Source: CAD feature listing. Evaluate the final solid. Frame: model axes, mm. Face numbers are marked on the shaded views. A direction names the side the tool comes from. Give positions to 0.01 mm unless a question says otherwise; leave off trailing zeros. Order: outer loops, then holes, each group sorted by start corner. A loop starts at its lowest first (then second) coordinate and runs counter-clockwise, first axis right, second up. Notation, with made-up numbers: (57.5, -25) -> (114.5, -25) arc R17 cw to (114.5, 5) -> close; hole circle Ø11 at (-16, -28). An arc over 180 degrees is marked (long way). Answer in a Markdown table with one row per item.
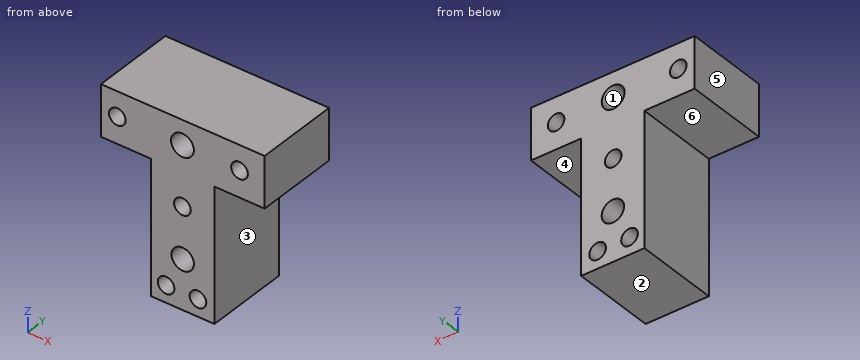
```python
from build123d import *

# Parameters (mm, degrees)
F0_R     = 2.413
F0_R_2   = 3.2512
F0_R_3   = 3.3147
F1_DEPTH = 24.384


with BuildPart() as f1:
    # F0 (on Front) → F1 (new body)
    with BuildSketch(Plane.XZ):
        Polygon((32.9184, 28.943862), (-14.5796, 28.943862), (-14.5796, 14.161062), (0, 14.161062), (0, -24.446938), (18.3388, -24.446938), (18.3388, 14.161062), (32.9184, 14.161062), align=None)
        with Locations((4.317999, -19.524282)):
            Circle(F0_R, mode=Mode.SUBTRACT)
        with Locations((9.143999, -10.159998)):
            Circle(F0_R_2, mode=Mode.SUBTRACT)
        with Locations((13.571819, -19.524282)):
            Circle(F0_R, mode=Mode.SUBTRACT)
        with Locations((9.0678, 4.570901)):
            Circle(F0_R, mode=Mode.SUBTRACT)
        with Locations((-9.830709, 21.781059)):
            Circle(F0_R, mode=Mode.SUBTRACT)
        with Locations((9.0678, 21.808036)):
            Circle(F0_R_3, mode=Mode.SUBTRACT)
        with Locations((25.6286, 21.781059)):
            Circle(F0_R, mode=Mode.SUBTRACT)
    extrude(amount=F1_DEPTH)


solid = f1.part
```
(1) Pull-direction query (X, two-part tool) for the marked faces 1, 2 and 3; classes: +X half, -X half, draft (parallel to the pull), parting line (faces both ways), or undercut.
A:
| item | result |
|---|---|
| face 1 | undercut |
| face 2 | draft |
| face 3 | +X half |
(2) Section query A-A (x = 13). Return the cut outline in (y, z), plus the area to 3 significant figures.
A:
| item | result |
|---|---|
| outline | (-24.38, -24.45) -> (0, -24.45) -> (0, -21.87) -> (-24.38, -21.87) -> close; (-24.38, -17.18) -> (0, -17.18) -> (0, 28.94) -> (-24.38, 28.94) -> close |
| area | 1,190 mm^2 |
(3) Ray query, probe 1 along Z at (x, y) = (9, -21.5); probe 2 along Z at (x, y) = (-10, -5.25); probe 3 along X at (y, z) = (-8, 20). Return the intervals inside material, ascending.
A:
| item | result |
|---|---|
| probe 1 | z = -24.45 to -13.41, -6.91 to 2.16, 6.98 to 18.49, 25.12 to 28.94 |
| probe 2 | z = 14.16 to 19.37, 24.19 to 28.94 |
| probe 3 | x = -14.58 to -11.46, -8.2 to 6.29, 11.85 to 24, 27.26 to 32.92 |
(4) Section query C-C (y = -19.5). Return the cut outline in (x, z), plus the area to 3 significant figures.
A:
| item | result |
|---|---|
| outline | (-14.58, 14.16) -> (0, 14.16) -> (0, -24.45) -> (18.34, -24.45) -> (18.34, 14.16) -> (32.92, 14.16) -> (32.92, 28.94) -> (-14.58, 28.94) -> close; hole circle Ø4.83 at (-9.83, 21.78); hole circle Ø4.83 at (4.32, -19.52); hole circle Ø6.63 at (9.07, 21.81); hole circle Ø6.5 at (9.14, -10.16); hole circle Ø4.83 at (9.07, 4.57); hole circle Ø4.83 at (13.57, -19.52); hole circle Ø4.83 at (25.63, 21.78) |
| area | 1,250 mm^2 |
(5) Access query for the marked faces 4, 5 and 6. Directions: +Z, -Z, +X, -X, +Y, -Y. A direction counts if a zero-diameter tool reaches every point of the face in a straight line with its end or side. Return the directions, or none.
A:
| item | result |
|---|---|
| face 4 | -Z, +X, +Y, -Y |
| face 5 | +Z, -Z, -X, +Y, -Y |
| face 6 | -Z, -X, +Y, -Y |
(6) Section query B-B (z = -11.5). Return the cut outline in (x, y), plus the area to 3 significant figures.
A:
| item | result |
|---|---|
| outline | (0, -24.38) -> (6.18, -24.38) -> (6.18, 0) -> (0, 0) -> close; (12.11, -24.38) -> (18.34, -24.38) -> (18.34, 0) -> (12.11, 0) -> close |
| area | 303 mm^2 |
(7) First-contact query: pin 1 Ø1 at (y, z) = (-12.5, -13) entering from +X; pin 2 Ø10 at (y, z) = (-10.5, -7.5) entering from -X; pin 3 Ø3 at (x, z) = (9.07, 4.57) entering from +Y; pin 4 Ø4.5 at (x, y) = (26.5, -17) entering from -Z. Flat tips, straight axial feed; report the tip coordinate or a pass-through.
A:
| item | result |
|---|---|
| pin 1 | stops at x = 18.34 |
| pin 2 | stops at x = 0 |
| pin 3 | passes through |
| pin 4 | stops at z = 14.16 |
(8) Section query D-D (x = -4). Return the cut outline in (y, z).
A:
| item | result |
|---|---|
| outline | (-24.38, 14.16) -> (0, 14.16) -> (0, 28.94) -> (-24.38, 28.94) -> close |
